Input: part model. Units: mm. Frame: model coordinates. Face numbers are marked on the shaded views. A direction names the side the tool comes from. Coordinates: 2 decimals unless noted, no trailing zeros. Loops run counter-clockwise (first coordinate to the right, second up) from the corner with the lowest first, then second, coordinate; pieces in that order, holes last.
(1) Section C-C, the plane y = -4. Return loops of the section in (x, z) (3 decimals), then the cut area to 3 significant figures.
(2) Contact query for flat-ended pins moving along their axis: P1, Ø2, axis at y = 0, z = -9, coming from the +X side; P2, Ø4, axis at x = 9, z = -5.5, coming from the -Y side; P3, Ø8, axis at x = -9.5, y = -3.5, coming from the -Z side. Output: stop coordinate, or through.
(3) Line query: L1, parallel to Y at x = -10, z = -6.75; L2, parallel to Y at x = 3.25, z = -7.75; L3, parallel to Z at x = -1.75, y = 0.5. Output: solid intervals per line, ascending.
(4) Set-up query: the marked faces 1, 2 and 3. Return all of +Z, -Z, +X, -X, +Y, -Y with unobstructed straight access to the full face (end or side cutting, diameter ignored); none if empty.
(5) Section B-B, the plane z = 0. Return loops of the section in (x, y) (3 decimals).
(6) Section D-D, the plane x = 3.5. Return loops of the section in (y, z), then the cut area to 3 significant figures.
(7) Section A-A, the plane x = 0. Return loops of the section in (y, z) (3 decimals), then the cut area to 3 significant figures.
```python
from build123d import *

# Parameters (mm, degrees)
F0_R     = 10.4
F1_DEPTH = 5
F0_R_2   = 12.7
F2_DEPTH = 3
F3_R     = 3.175
F4_DEPTH = 7


with BuildPart() as f1:
    # F0 (on Front) → F1 (new body)
    with BuildSketch(Plane.XZ):
        Circle(F0_R)
    extrude(amount=-F1_DEPTH)

    # F0 (on Front) → F2 (join)
    with BuildSketch(Plane.XZ):
        Circle(F0_R_2)
        Circle(F0_R, mode=Mode.SUBTRACT)
        Circle(F0_R)
    extrude(amount=F2_DEPTH)

    # F3 (on face) → F4 (join)
    with BuildSketch(Plane.XZ.offset(3)):
        Circle(F3_R)
    extrude(amount=F4_DEPTH)


solid = f1.part
```
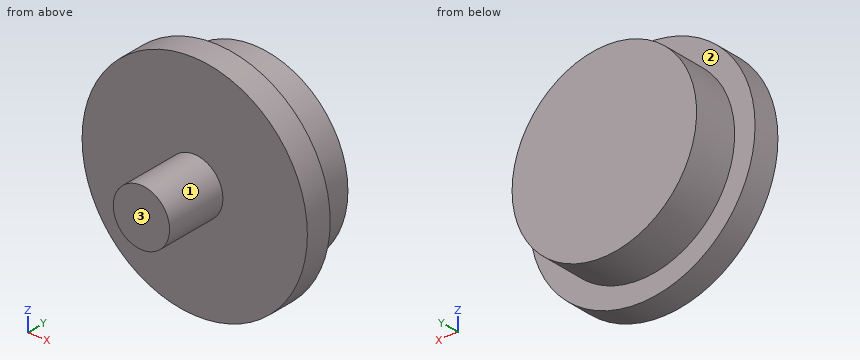
Report:
1. outline: circle Ø6.35 at (0, 0)
1. area: 31.7 mm2
2. P1: stops at x = 9.86
2. P2: stops at y = -3
2. P3: stops at z = -11.43
3. L1: y = -3 to 0
3. L2: y = -3 to 5
3. L3: z = -10.25 to 10.25
4. face 1: -Y
4. face 2: +Y
4. face 3: +Z, -Z, +X, -X, -Y
5. outline: (-12.7, -3) - (-3.175, -3) - (-3.175, -10) - (3.175, -10) - (3.175, -3) - (12.7, -3) - (12.7, 0) - (10.4, 0) - (10.4, 5) - (-10.4, 5) - (-10.4, 0) - (-12.7, 0) - close
6. outline: (-3, -12.21) - (0, -12.21) - (0, -9.79) - (5, -9.79) - (5, 9.79) - (0, 9.79) - (0, 12.21) - (-3, 12.21) - close
6. area: 171 mm2
7. outline: (-10, -3.175) - (-3, -3.175) - (-3, -12.7) - (0, -12.7) - (0, -10.4) - (5, -10.4) - (5, 10.4) - (0, 10.4) - (0, 12.7) - (-3, 12.7) - (-3, 3.175) - (-10, 3.175) - close
7. area: 225 mm2
